Design review of the part built by this model. Coordinates are the model's own, in mm. Face numbers are marked on the shaded views. A direction names the side the tool comes from. Give positions to 0.01 mm unless a question says otherwise; leave off trailing zeros. Loops run counter-clockwise (first coordinate to the right, second up) from the corner with the lowest first, then second, coordinate; pieces in that order, holes last. Notation, with made-up numbers: (-10.5, -4.5) -> (7.5, -4.5) arc R5 cw to (7.5, 3.5) -> close; hole circle Ø3 at (10.25, 63). An arc over 180 degrees is marked (long way). Answer in a Markdown table with one row per item. Add a question column.
(1) Consider section A-A on y = -41.5. Write out the cut boundary in (x, z).
(2) Consider section C-C on x = 104.5. Write out the cut boundary in (y, z).
(3) Draft analysis for pull direction Y (two halves, no side actions). For the marked faces 4, 5 and 6, state which applies: +Y half, -Y half, draft (parallel to the pull), parting line (faces both ways), or undercut.
(4) For pin 1 (9.5 mm diameter, centred on x = 126.5, z = -18, fed in from -Y); pin 2 (17.5 mm diameter, centred on x = 118, z = -15, fed in from +Y); pin 3 (6 mm diameter, centred on y = -50, z = -8.5, fed in from +X); pin 4 (4 mm diameter, centred on y = -26.5, z = -24.5, fed in from -X), all flat-tipped, find the tip position at first contact; note any pin that passes through.
(5) Consider section D-D on y = -47.5. Write out the cut boundary in (x, z), then the cut area to 3 significant figures.
(6) For the marked faces 1, 2 and 3, list the 3-axis set-ups (+Z, -Z, +X, -X, +Y, -Y) from which the entire face can be reached by the end or side of a thin tool; tool diameter is ignored.
(7) Consider section B-B on y = -35.5. Write out the cut boundary in (x, z).
(8) For line 1 (Z direction, x = 58.5, y = -42); line 2 (Y direction, x = 102, z = -21.5); line 3 (Y direction, x = 45.5, z = -2), list the stretches that pass through material, from the lowest coordinate up.
from build123d import *

# Parameters (mm, degrees)
EXTRUDE_1_DEPTH          = 35
CUT_EXTRUDE_1_DEPTH      = 185.022712326
SKETCH_3_W               = 23
SKETCH_3_H               = 16.98
CUT_EXTRUDE_2_DEPTH      = 159.069540958
SKETCH_5_W               = 23
SKETCH_5_H               = 7.5
CUT_EXTRUDE_3_DEPTH      = 5
SKETCH_6_R               = 1.5
CUT_EXTRUDE_4_DEPTH      = 138.067283793
MIRROR_2_COPY_1_SKETCH_W = 23
MIRROR_2_COPY_1_SKETCH_H = 7.5
MIRROR_2_COPY_1_DEPTH    = 5
MIRROR_2_COPY_2_SKETCH_R = 1.5
MIRROR_2_COPY_2_DEPTH    = 138.067283793
FILLET_3_R               = 2
SKETCH_7_R               = 1.5
CUT_EXTRUDE_5_DEPTH      = 8


with BuildPart() as part:
    # 草图1 → 凸台-拉伸1 (new body)
    with BuildSketch(Plane.XY):
        with BuildLine():
            ThreePointArc((40.282032616, -21.905575199), (41.494272902, -22.715568261), (42.924207815, -23))
            Line((42.924207815, -23), (158.071347708, -23))
            ThreePointArc((158.071347708, -23), (159.501282621, -22.715568261), (160.713522906, -21.905575199))
            Line((160.713522906, -21.905575199), (169.40335296, -13.215745145))
            Line((169.40335296, -13.215745145), (169.40335296, -59.784254855))
            Line((169.40335296, -59.784254855), (160.713522906, -51.094424801))
            ThreePointArc((160.713522906, -51.094424801), (159.501282621, -50.284431739), (158.071347708, -50))
            Line((158.071347708, -50), (42.924207815, -50))
            ThreePointArc((42.924207815, -50), (41.494272902, -50.284431739), (40.282032616, -51.094424801))
            Line((40.282032616, -51.094424801), (28.592202563, -62.784254855))
            Line((28.592202563, -62.784254855), (28.592202563, -10.215745145))
            Line((28.592202563, -10.215745145), (40.282032616, -21.905575199))
        make_face()
    extrude(amount=-EXTRUDE_1_DEPTH)

    # 草图2 → 切除-拉伸1 (cut, through all)
    with BuildSketch(Plane.XY):
        with BuildLine():
            Line((40.282032616, -21.905575199), (28.592202563, -10.215745145))
            Line((28.592202563, -10.215745145), (28.592202563, -62.784254855))
            Line((28.592202563, -62.784254855), (40.282032616, -51.094424801))
            ThreePointArc((40.282032616, -51.094424801), (41.494272902, -50.284431739), (42.924207815, -50))
            Line((42.924207815, -50), (158.071347708, -50))
            ThreePointArc((158.071347708, -50), (159.501282621, -50.284431739), (160.713522906, -51.094424801))
            Line((160.713522906, -51.094424801), (169.40335296, -59.784254855))
            Line((169.40335296, -59.784254855), (169.40335296, -13.215745145))
            Line((169.40335296, -13.215745145), (160.713522906, -21.905575199))
            ThreePointArc((160.713522906, -21.905575199), (159.501282621, -22.715568261), (158.071347708, -23))
            Line((158.071347708, -23), (42.924207815, -23))
            ThreePointArc((42.924207815, -23), (41.494272902, -22.715568261), (40.282032616, -21.905575199))
        make_face()
        with BuildLine():
            Line((28.602202563, -10.239887281), (28.602202563, -62.760112719))
            Line((28.602202563, -62.760112719), (40.274961549, -51.087353734))
            ThreePointArc((40.274961549, -51.087353734), (41.490446067, -50.275192944), (42.924207815, -49.99))
            Line((42.924207815, -49.99), (158.071347708, -49.99))
            ThreePointArc((158.071347708, -49.99), (159.505109455, -50.275192944), (160.720593974, -51.087353734))
            Line((160.720593974, -51.087353734), (169.39335296, -59.760112719))
            Line((169.39335296, -59.760112719), (169.39335296, -13.239887281))
            Line((169.39335296, -13.239887281), (160.720593974, -21.912646266))
            ThreePointArc((160.720593974, -21.912646266), (159.505109455, -22.724807057), (158.071347708, -23.01))
            Line((158.071347708, -23.01), (42.924207815, -23.01))
            ThreePointArc((42.924207815, -23.01), (41.490446067, -22.724807057), (40.274961549, -21.912646266))
            Line((40.274961549, -21.912646266), (28.602202563, -10.239887281))
        make_face(mode=Mode.SUBTRACT)
    extrude(amount=-CUT_EXTRUDE_1_DEPTH, mode=Mode.SUBTRACT)

    # 草图3 → 切除-拉伸2 (cut, through all)
    with BuildSketch(Plane(origin=(169.39335296, 0, 0), x_dir=(0, 0, -1), z_dir=(1, 0, 0))):
        with Locations((17.5, -36.5)):
            Rectangle(SKETCH_3_W, SKETCH_3_H)
    extrude(amount=-CUT_EXTRUDE_2_DEPTH, mode=Mode.SUBTRACT)

    # 草图5 → 切除-拉伸3 (cut)
    with BuildSketch(Plane(origin=(36.796101281, -36.796101281, 0), x_dir=(0, 0, -1), z_dir=(0.7071067811865873, -0.7071067811865078, 0))):
        with Locations((17.5, -15.337922697)):
            Rectangle(SKETCH_5_W, SKETCH_5_H)
        with Locations((17.5, -7.837922697)):
            Rectangle(SKETCH_5_W, SKETCH_5_H)
    cut_extrude_3 = extrude(amount=CUT_EXTRUDE_3_DEPTH, mode=Mode.SUBTRACT)

    # 草图6 → 切除-拉伸4 (cut, through all)
    with BuildSketch(Plane(origin=(40.331635187, -40.331635187, 0), x_dir=(0, 0, 1), z_dir=(-0.7071067811865871, 0.707106781186508, 0))):
        with Locations(Location((-12, -13.587922697, 0), (0, 0, 270))):
            Circle(SKETCH_6_R)
        with Locations(Location((-22, -13.587922697, 0), (0, 0, 270))):
            Circle(SKETCH_6_R)
    cut_extrude_4 = extrude(amount=-CUT_EXTRUDE_4_DEPTH, mode=Mode.SUBTRACT)

    # 镜向1: 切除-拉伸3, 切除-拉伸4 across plane
    add(cut_extrude_3.mirror(Plane.ZX.offset(-36.5)), mode=Mode.SUBTRACT)
    add(cut_extrude_4.mirror(Plane.ZX.offset(-36.5)), mode=Mode.SUBTRACT)

    # 镜向2: 切除-拉伸3, 切除-拉伸4 across plane
    add(cut_extrude_3.mirror(Plane(origin=(98.997777761, 0, 0), x_dir=(0, 0, 1), z_dir=(1, 0, 0))), mode=Mode.SUBTRACT)
    add(cut_extrude_4.mirror(Plane(origin=(98.997777761, 0, 0), x_dir=(0, 0, 1), z_dir=(1, 0, 0))), mode=Mode.SUBTRACT)

    # 镜向2 copy 1 sketch → 镜向2 copy 1 (cut)
    with BuildSketch(Plane(origin=(161.199454241, -36.203898719, 0), x_dir=(0, 0, -1), z_dir=(-0.7071067811865942, 0.7071067811865009, 0))):
        with Locations((17.5, -15.337922697)):
            Rectangle(MIRROR_2_COPY_1_SKETCH_W, MIRROR_2_COPY_1_SKETCH_H)
        with Locations((17.5, -7.837922697)):
            Rectangle(MIRROR_2_COPY_1_SKETCH_W, MIRROR_2_COPY_1_SKETCH_H)
    extrude(amount=MIRROR_2_COPY_1_DEPTH, mode=Mode.SUBTRACT)

    # 镜向2 copy 2 sketch → 镜向2 copy 2 (cut, through all)
    with BuildSketch(Plane(origin=(157.663920335, -32.668364813, 0), x_dir=(0, 0, 1), z_dir=(0.707106781186594, -0.7071067811865012, 0))):
        with Locations(Location((-12, -13.587922697, 0), (0, 0, 270))):
            Circle(MIRROR_2_COPY_2_SKETCH_R)
        with Locations(Location((-22, -13.587922697, 0), (0, 0, 270))):
            Circle(MIRROR_2_COPY_2_SKETCH_R)
    extrude(amount=-MIRROR_2_COPY_2_DEPTH, mode=Mode.SUBTRACT)

    # 圆角3
    fillet_3_edges = [part.edges().sort_by_distance(p)[0] for p in [
        (98.997777761, -44.99, -6),
        (98.997777761, -44.99, -29),
        (98.997777761, -28.01, -6),
        (98.997777761, -28.01, -29),
        (169.39335296, -13.239887281, -17.5),
        (169.39335296, -59.760112719, -17.5),
        (28.602202563, -62.760112719, -17.5),
        (28.602202563, -10.239887281, -17.5),
    ]]
    fillet(fillet_3_edges, radius=FILLET_3_R)

    # 草图7 → 切除-拉伸5 (cut)
    with BuildSketch(Plane.XY):
        with Locations((165.39335296, -41.5)):
            Circle(SKETCH_7_R)
        with Locations((165.39335296, -31.5)):
            Circle(SKETCH_7_R)
    extrude(amount=-CUT_EXTRUDE_5_DEPTH, mode=Mode.SUBTRACT)


solid = part.part
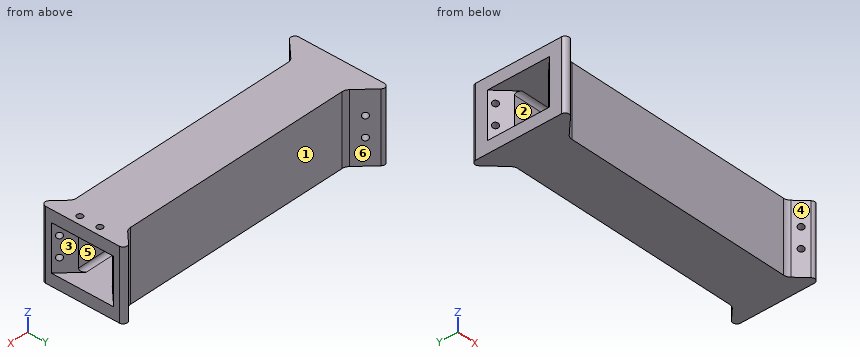
Values follow:
| question | item | result |
|---|---|---|
| 1 | outline | (28.6, -35) -> (169.39, -35) -> (169.39, -29) -> (28.6, -29) -> close; (28.6, -6) -> (163.89, -6) -> (163.89, 0) -> (28.6, 0) -> close; (166.89, -6) -> (169.39, -6) -> (169.39, 0) -> (166.89, 0) -> close |
| 2 | outline | (-49.99, -35) -> (-23.01, -35) -> (-23.01, 0) -> (-49.99, 0) -> close; hole (-44.99, -27) arc R2 ccw to (-42.99, -29) -> (-30.01, -29) arc R2 ccw to (-28.01, -27) -> (-28.01, -8) arc R2 ccw to (-30.01, -6) -> (-42.99, -6) arc R2 ccw to (-44.99, -8) -> close |
| 3 | face 4 | -Y half |
| 3 | face 5 | undercut |
| 3 | face 6 | +Y half |
| 4 | pin 1 | y = -49.99 |
| 4 | pin 2 | y = -23.01 |
| 4 | pin 3 | x = 169.39 |
| 4 | pin 4 | x = 32.16 |
| 5 | outline | (28.6, -35) -> (169.39, -35) -> (169.39, -29) -> (164.83, -29) -> (164.83, -6) -> (169.39, -6) -> (169.39, 0) -> (28.6, 0) -> (28.6, -6) -> (33.16, -6) -> (33.16, -29) -> (28.6, -29) -> close |
| 5 | area | 4,720 mm2 |
| 6 | face 1 | +Z, -Z, +Y |
| 6 | face 2 | +X, -X |
| 6 | face 3 | +X |
| 7 | outline | (28.6, -35) -> (169.39, -35) -> (169.39, -29) -> (28.6, -29) -> close; (28.6, -6) -> (169.39, -6) -> (169.39, 0) -> (28.6, 0) -> close |
| 8 | line 1 | -35 to -29, -6 to 0 |
| 8 | line 2 | -49.99 to -44.99, -28.01 to -23.01 |
| 8 | line 3 | -49.99 to -23.01 |
